Here's the drawing with two shaded views (mm, measured from the low corner). I have some questions. A direction names the side the tool comes from. Give positions to 0.01 mm unless a question says otherwise; leave off trailing zeros. Write each loop counter-clockwise with the first axis right and the second up, starting at its lowest first coordinate (ties: lowest second). Pieces come first, ordered by that corner, then holes.
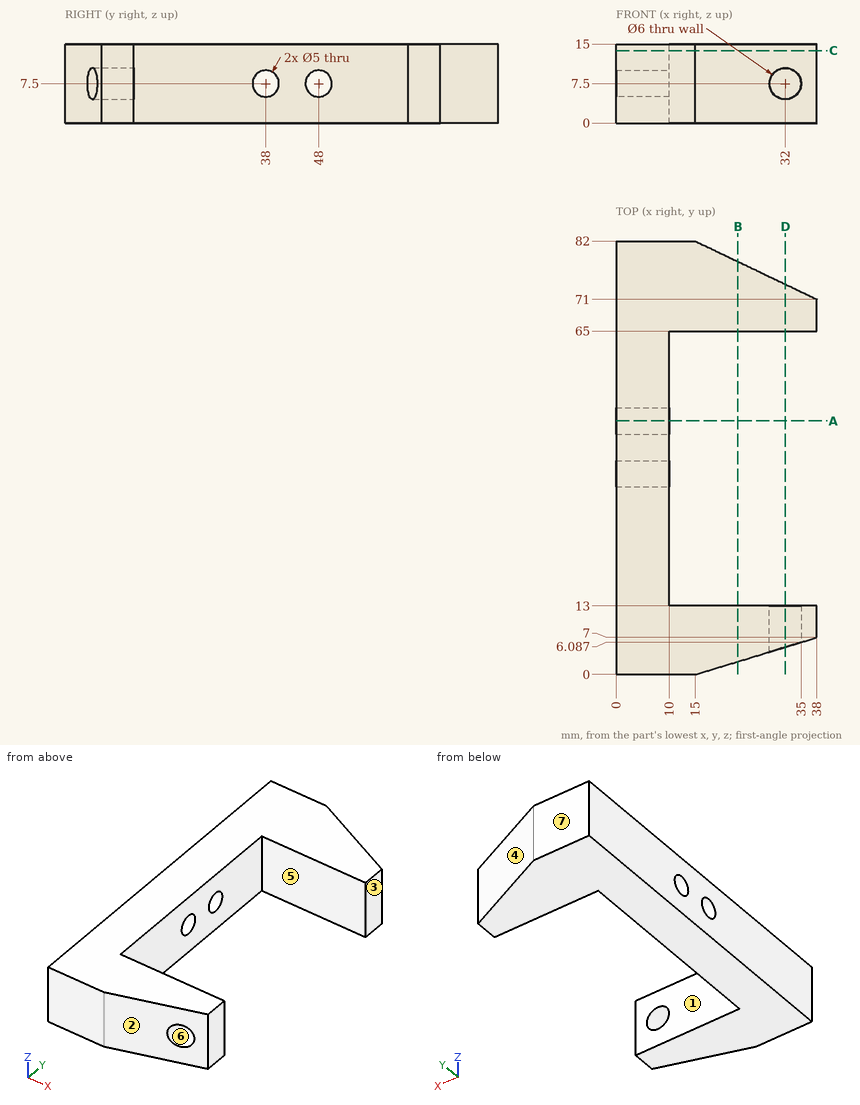
(1) For the marked faces 5, 6 and 7, which set-ups out of +Z, -Z, +X, -X, +Y, -Y let a thin tool reach every point of the face, with its end or its side?
Returned:
face 5: +Z, -Z, +X
face 6: -Y
face 7: +Z, -Z, +X, -X, +Y
(2) Imagine slicing it at C-C, the plane z = 13.75. Write out the boundary of the cut face in (x, y), plus the area to 3 significant figures.
Returned:
outline: (0, 0) - (15, 0) - (38, 7) - (38, 13) - (10, 13) - (10, 65) - (38, 65) - (38, 71) - (15, 82) - (0, 82) - close
area: 1,450 mm2
(3) Imagine slicing it at B-B, the plane x = 23. Write out the boundary of the cut face in (y, z), plus the area to 3 significant figures.
Returned:
outline: (2.43, 0) - (13, 0) - (13, 15) - (2.43, 15) - close; (65, 0) - (78.17, 0) - (78.17, 15) - (65, 15) - close
area: 356 mm2
(4) Imagine slicing it at D-D, the plane x = 32. Write out the boundary of the cut face in (y, z), plus the area to 3 significant figures.
Returned:
outline: (5.17, 0) - (13, 0) - (13, 4.5) - (5.17, 4.5) - close; (5.17, 10.5) - (13, 10.5) - (13, 15) - (5.17, 15) - close; (65, 0) - (73.87, 0) - (73.87, 15) - (65, 15) - close
area: 203 mm2
(5) If we mould it in two halves opening along Y, with no side actions, what happens to the marked faces 1, 2, 3 and 4? For each: +Y half, -Y half, draft (parallel to the pull), parting line (faces both ways), or undercut.
Returned:
face 1: undercut
face 2: -Y half
face 3: draft
face 4: +Y half
(6) Will these pins go through, and if not, where does the flat tip stop? P1, Ø7, axis at x = 32, z = 7.5, coming from the +Y side; P2, Ø5, axis at x = 23, z = 3, coming from the -Y side; P3, Ø1.5, axis at y = 30, z = 8.5, coming from the +X side; P4, Ø4, axis at y = 38, z = 7.5, coming from the -X side.
Returned:
P1: stops at y = 75.54
P2: stops at y = 1.67
P3: stops at x = 10
P4: passes through
(7) If I drill on L1, parallel to Y at x = 2.25, z = 7.5; L2, parallel to Y at x = 14, z = 8.5; L3, parallel to X at y = 35, z = 9.75, over which ranges is the centre line in solid material (lowest first)?
Returned:
L1: y = 0 to 35.5, 40.5 to 45.5, 50.5 to 82
L2: y = 0 to 13, 65 to 82
L3: x = 0 to 10
(8) Imagine slicing it at A-A, the plane y = 48. Write out the boundary of the cut face in (x, z), plus the area to 3 significant figures.
Returned:
outline: (0, 0) - (10, 0) - (10, 5) - (0, 5) - close; (0, 10) - (10, 10) - (10, 15) - (0, 15) - close
area: 100 mm2
